from build123d import *

# Parameters (mm, degrees)
ESQUISSE1_W             = 70
ESQUISSE1_H             = 70
BOSS_EXTRU_1_DEPTH      = 90
BOSS_EXTRU_2_DEPTH      = 5
BOSS_EXTRU_2_DEPTH_BACK = 5
ESQUISSE2_R             = 7.5


with BuildPart() as part:
    # Esquisse1 → Boss.-Extru.1 (new body)
    with BuildSketch(Plane.XY):
        Rectangle(ESQUISSE1_W, ESQUISSE1_H)
    extrude(amount=BOSS_EXTRU_1_DEPTH)

    # Esquisse2 → Boss.-Extru.2 (add, two sides: drawn at the far end of the back side and taken through both)
    with BuildSketch(Plane(origin=(0, 0, 0), x_dir=(0, 0, -1), z_dir=(1, 0, 0)).offset(-BOSS_EXTRU_2_DEPTH_BACK)):
        with BuildLine():
            Line((-57.5, 35), (-57.5, 65))
            ThreePointArc((-57.5, 65), (-45, 77.5), (-32.5, 65))
            Line((-32.5, 65), (-32.5, 35))
            Line((-32.5, 35), (-57.5, 35))
        make_face()
        with Locations((-45, 65)):
            Circle(ESQUISSE2_R, mode=Mode.SUBTRACT)
    extrude(amount=BOSS_EXTRU_2_DEPTH + BOSS_EXTRU_2_DEPTH_BACK)


solid = part.part
Verification items for the finished model (mm, model axes). A direction names the side the tool comes from. Coordinates: 2 decimals unless noted, no trailing zeros. Order: outer loops, then holes, each group sorted by start corner. A loop starts at its lowest first (then second) coordinate and runs counter-clockwise, first axis right, second up.
Item 1: Section check C-C, the plane y = 71. Enter the section's corners in (x, z), then the cut area to 3 significant figures.
Filled in:
outline: (-5, 34.03) - (5, 34.03) - (5, 40.5) - (-5, 40.5) - close; (-5, 49.5) - (5, 49.5) - (5, 55.97) - (-5, 55.97) - close
area: 129 mm2
Item 2: Access from +Z, -Z, +X, -X, +Y, -Y to the whole of each face (thin tool, end or side, straight path). Record for faces 4 (the face through (-5, 52, 45)), 5 (the face through (5, 52, 45)), 6 (the face through (0, 50, 57.5)).
Filled in:
face 4: +Z, -Z, -X, +Y
face 5: +Z, -Z, +X, +Y
face 6: +Z, +X, -X, +Y
Item 3: Release check for a two-part mould opening along Y. For faces 1 (the face through (0, -35, 44)), 2 (the face through (-35, 0, 44)), 3 (the face through (-0.07, 67.253, 37.846)) record: +Y half, -Y half, draft (parallel to the pull), parting line (faces both ways), or undercut.
Filled in:
face 1: -Y half
face 2: draft
face 3: undercut
Item 4: Material ranges on L1, parallel to Y at x = 1.5, z = 45; L2, parallel to Y at x = -12, z = 73.5; L3, parallel to Z at x = 0.5, y = 60, recorded low to high.
Filled in:
L1: y = -35 to 57.5, 72.5 to 77.5
L2: y = -35 to 35
L3: z = 32.5 to 39.41, 50.59 to 57.5
Item 5: Section check B-B, the plane x = 0.5. Enter the section's corners in (y, z), then the cut area to 3 significant figures.
Filled in:
outline: (-35, 0) - (35, 0) - (35, 32.5) - (65, 32.5) arc R12.5 ccw to (65, 57.5) - (35, 57.5) - (35, 90) - (-35, 90) - close; hole circle Ø15 at (65, 45)
area: 7,120 mm2
Item 6: Depth check by flat-ended pin: pin 1 (7.5 mm diameter, centred on y = 47, z = 48.5, fed in from +X); pin 2 (21 mm diameter, centred on x = -3, z = 32.5, fed in from +Y); pin 3 (13.5 mm diameter, centred on y = 65, z = 45, fed in from -X); pin 4 (3 mm diameter, centred on x = 0.5, y = 57.5, fed in from -Z). Enter the tip coordinate at first touch or a pass-through.
Filled in:
pin 1: stops at x = 5
pin 2: stops at y = 77.34
pin 3: passes through
pin 4: stops at z = 32.5
Item 7: Section check D-D, the plane y = 48. Enter the section's corners in (x, z), then the cut area to 3 significant figures.
Filled in:
outline: (-5, 32.5) - (5, 32.5) - (5, 57.5) - (-5, 57.5) - close
area: 250 mm2
Item 8: Section check A-A, the plane z = 45. Enter the section's corners in (x, y).
Filled in:
outline: (-35, -35) - (35, -35) - (35, 35) - (5, 35) - (5, 57.5) - (-5, 57.5) - (-5, 35) - (-35, 35) - close; (-5, 72.5) - (5, 72.5) - (5, 77.5) - (-5, 77.5) - close
